from build123d import *

# Parameters (mm, degrees)
SKETCH_W        = 104
SKETCH_H        = 62
PAD_DEPTH       = 6.5
SKETCH001_W     = 101.5
SKETCH001_H     = 59.5
POCKET_DEPTH    = 4
SKETCH002_W     = 50
SKETCH002_H     = 1.5
POCKET001_DEPTH = 0.6
SKETCH003_W     = 50
SKETCH003_H     = 1.5
POCKET002_DEPTH = 0.6
FILLET_R        = 0.75
SKETCH004_R     = 2.5
POCKET003_DEPTH = 3


with BuildPart() as part:
    # Sketch → Pad (new body)
    with BuildSketch(Plane.XY):
        Rectangle(SKETCH_W, SKETCH_H)
    extrude(amount=PAD_DEPTH)

    # Sketch001 (on Face6 of Pad) → Pocket (cut)
    with BuildSketch(Plane.XY.offset(6.5)):
        Rectangle(SKETCH001_W, SKETCH001_H)
    extrude(amount=-POCKET_DEPTH, mode=Mode.SUBTRACT)

    # Sketch002 (on Face7 of Pocket) → Pocket001 (cut)
    with BuildSketch(Plane.XZ.offset(-29.75)):
        with Locations((0, 4.5)):
            Rectangle(SKETCH002_W, SKETCH002_H)
    extrude(amount=-POCKET001_DEPTH, mode=Mode.SUBTRACT)

    # Sketch003 (on Face9 of Pocket001) → Pocket002 (cut)
    with BuildSketch(Plane(origin=(0, -29.75, 0), x_dir=(-1, 0, 0), z_dir=(0, 1, 0))):
        with Locations((0, 4.5)):
            Rectangle(SKETCH003_W, SKETCH003_H)
    extrude(amount=-POCKET002_DEPTH, mode=Mode.SUBTRACT)

    # Fillet
    fillet_edges = [part.edges().sort_by_distance(p)[0] for p in [
        (0, -31, 0),
        (52, 0, 0),
        (0, 31, 0),
        (-52, 0, 0),
    ]]
    fillet(fillet_edges, radius=FILLET_R)

    # Sketch004 (on Face15 of Fillet) → Pocket003 (cut)
    with BuildSketch(Plane.XY.offset(2.5)):
        with Locations((-45, -25)):
            Circle(SKETCH004_R)
    extrude(amount=-POCKET003_DEPTH, mode=Mode.SUBTRACT)


solid = part.part
Verification items for the finished model (mm, model axes). A direction names the side the tool comes from. Coordinates: 2 decimals unless noted, no trailing zeros. Order: outer loops, then holes, each group sorted by start corner. A loop starts at its lowest first (then second) coordinate and runs counter-clockwise, first axis right, second up. Notation, with made-up numbers: M 20.5,61.5 L 29.5,61.5 A16 cw 29.5,87.5 Z; hole C 41,48 d6. An arc over 180 degrees is marked long. One line per item, written item: value. Start each with the question number.
Item 1: Sectioned sample at A-A on x = -45. Record the cut outline in (y, z), then the cut area to 3 significant figures.
Item 2: Sectioned sample at D-D on y = 5. Record the cut outline in (x, z), then the cut area to 3 significant figures.
Item 3: Sectioned sample at C-C on x = 11. Record the cut outline in (y, z), then the cut area to 3 significant figures.
Item 4: Thickness scan on probe 1 along Y at (x, z) = (-45, 0.9); probe 2 along X at (y, z) = (12, 5.25); probe 3 along Y at (x, z) = (-7.5, 5.5). Record the ranges inside material, lowest first.
Item 5: Mould release check, pull along Y, two halves, no side actions. Record for faces 3 (the flat face through (-50.75, 0, 5)), 4 (the flat face through (-1, 0, 0)), 5 (the flat face through (-1, 31, 4)), 6 (the cylindrical face through (-43.66, -22.89, 1.27)): pulls with the +Y half, pulls with the -Y half, needs draft (parallel to the pull), parting line crosses it, or undercut.
Item 6: Sectioned sample at B-B on y = -25. Record the cut outline in (x, z).
Item 7: Depth check by flat-ended pin: P1, Ø12, axis at x = -14, y = 22, coming from the +Z side. Enter the tip coordinate at first touch or a pass-through.
Item 8: Access from +Z, -Z, +X, -X, +Y, -Y to the whole of each face (thin tool, end or side, straight path). Record for faces 1 (the flat face through (-1, 0, 2.5)), 2 (the flat face through (52, 0, 4)).
Calculated:
1. outline: M -31,0.75 A0.75 ccw -30.25,0 L -27.5,0 L -27.5,2.5 L -29.75,2.5 L -29.75,6.5 L -31,6.5 Z; M -22.5,0 L 30.25,0 A0.75 ccw 31,0.75 L 31,6.5 L 29.75,6.5 L 29.75,2.5 L -22.5,2.5 Z
1. area: 152 mm^2
2. outline: M -52,0.75 A0.75 ccw -51.25,0 L 51.25,0 A0.75 ccw 52,0.75 L 52,6.5 L 50.75,6.5 L 50.75,2.5 L -50.75,2.5 L -50.75,6.5 L -52,6.5 Z
2. area: 270 mm^2
3. outline: M -31,0.75 A0.75 ccw -30.25,0 L 30.25,0 A0.75 ccw 31,0.75 L 31,6.5 L 29.75,6.5 L 29.75,5.25 L 30.35,5.25 L 30.35,3.75 L 29.75,3.75 L 29.75,2.5 L -29.75,2.5 L -29.75,3.75 L -30.35,3.75 L -30.35,5.25 L -29.75,5.25 L -29.75,6.5 L -31,6.5 Z
3. area: 163 mm^2
4. probe 1: -31 to -27.5, -22.5 to 31
4. probe 2: -52 to -50.75, 50.75 to 52
4. probe 3: -31 to -29.75, 29.75 to 31
5. face 3: undercut
5. face 4: needs draft
5. face 5: pulls with the +Y half
5. face 6: undercut
6. outline: M -52,0.75 A0.75 ccw -51.25,0 L -47.5,0 L -47.5,2.5 L -50.75,2.5 L -50.75,6.5 L -52,6.5 Z; M -42.5,0 L 51.25,0 A0.75 ccw 52,0.75 L 52,6.5 L 50.75,6.5 L 50.75,2.5 L -42.5,2.5 Z
7. P1: z = 2.5
8. face 1: +Z
8. face 2: +Z, -Z, +X, +Y, -Y
